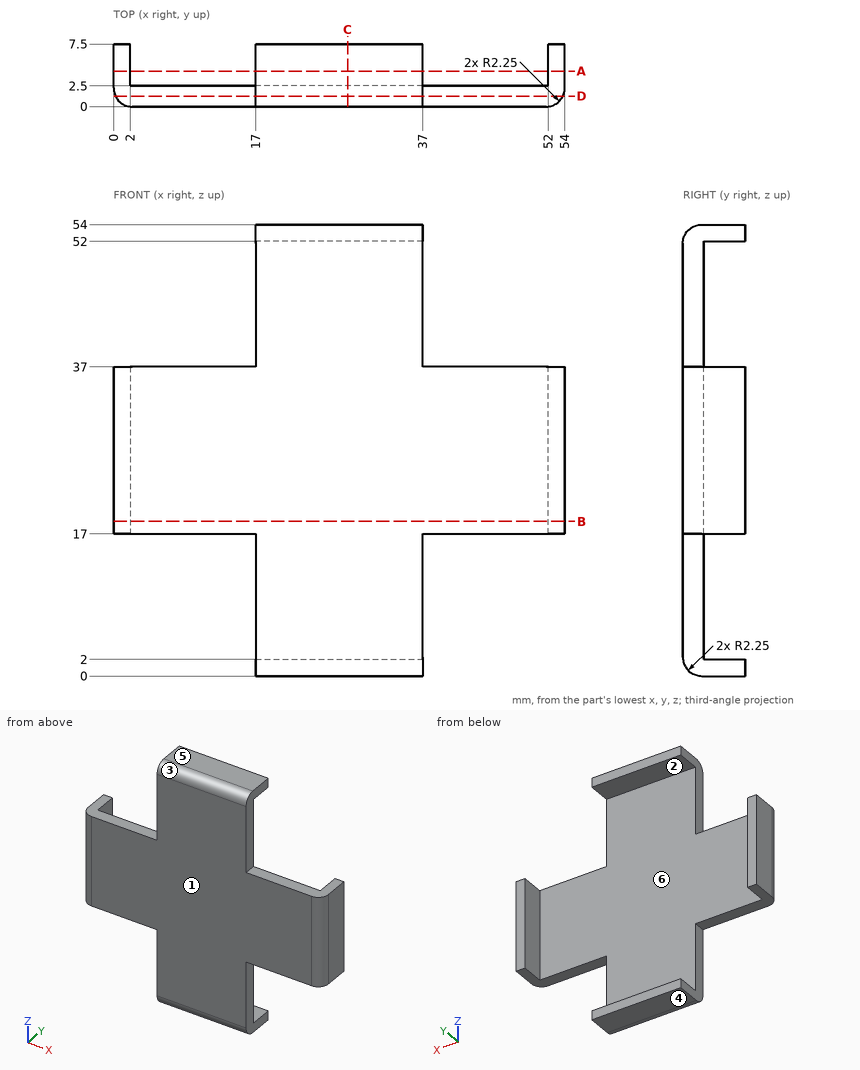
Part print with two shaded views. Sizes in mm from the minimum x, y, z corner. A direction names the side the tool comes from. Coordinates: 2 decimals unless noted, no trailing zeros. Write each loop counter-clockwise with the first axis right and the second up, starting at its lowest first coordinate (ties: lowest second). Pieces come first, ordered by that corner, then holes. Notation, with made-up numbers: (70.5, -4.75) - (124.5, -4.75) arc R24 ccw to (124.5, 33.25) - close; hole circle Ø1 at (-35.75, 30.5). An arc over 180 degrees is marked (long way). Put each result on its own line as item: value.
1. 3-axis set-ups, long thin cutter, end or side, ignore diameter. For the marked faces 5 and 6: which of +Z, -Z, +X, -X, +Y, -Y reach the whole face in a straight line?
Final values:
face 5: +Z, +X, -X, +Y, -Y
face 6: +Y
2. Probe line 1 along X through (y, z) = (7, 27.5); line 2 along Y through (x, z) = (41, 29). List the from-to ranges inside material, lowest first. Write a range as [from, to].
Final values:
line 1: x = [0, 2], [52, 54]
line 2: y = [0, 2.5]
3. Flat gauge pins, fed straight in: pin 1 Ø1 at (x, z) = (29, 48.5) entering from +Y; pin 2 Ø2 at (y, z) = (2, 40) entering from -X. Where does each tip first touch, or does it go through?
Final values:
pin 1: stops at y = 2.5
pin 2: stops at x = 17
4. Band-saw the part on A-A (y = 4.25). Write the cut outline in (x, z).
Final values:
outline: (0, 17) - (2, 17) - (2, 37) - (0, 37) - close; (17, 0) - (37, 0) - (37, 2) - (17, 2) - close; (17, 52) - (37, 52) - (37, 54) - (17, 54) - close; (52, 17) - (54, 17) - (54, 37) - (52, 37) - close
5. Two-plate mould, pull along Z, no slides. Class the marked faces 1, 2, 3 and 4: +Z half, -Z half, draft (parallel to the pull), parting line (faces both ways), or undercut.
Final values:
face 1: draft
face 2: undercut
face 3: +Z half
face 4: -Z half
6. Band-saw the part on B-B (z = 18.5). Write the cut outline in (x, y).
Final values:
outline: (0, 2.25) arc R2.25 ccw to (2.25, 0) - (51.75, 0) arc R2.25 ccw to (54, 2.25) - (54, 7.5) - (52, 7.5) - (52, 2.5) - (2, 2.5) - (2, 7.5) - (0, 7.5) - close
7. Band-saw the part on D-D (y = 1.25). Write the cut outline in (x, z), then the cut area to 3 significant figures.
Final values:
outline: (0.23, 17) - (17, 17) - (17, 0.23) - (37, 0.23) - (37, 17) - (53.77, 17) - (53.77, 37) - (37, 37) - (37, 53.77) - (17, 53.77) - (17, 37) - (0.23, 37) - close
area: 1,740 mm²
8. Band-saw the part on C-C (x = 28). Write the cut outline in (y, z).
Final values:
outline: (0, 2.25) arc R2.25 ccw to (2.25, 0) - (7.5, 0) - (7.5, 2) - (2.5, 2) - (2.5, 52) - (7.5, 52) - (7.5, 54) - (2.25, 54) arc R2.25 ccw to (0, 51.75) - close
